For this review, use the dimensioned drawing (mm, ordinates from the lowest corner) and the shaded views. Give positions to 0.01 mm unless a question says otherwise; leave off trailing zeros. Loops run counter-clockwise (first coordinate to the right, second up) from the corner with the lowest first, then second, coordinate; pieces in that order, holes last. Notation, with made-up numbers: M 11.5,-28.75 L 35.5,-28.75 A29 cw 35.5,5.25 Z; hole C 38.5,10.25 d10. An arc over 180 degrees is marked long. Use CSV: the item, a comma, the result in double quotes.
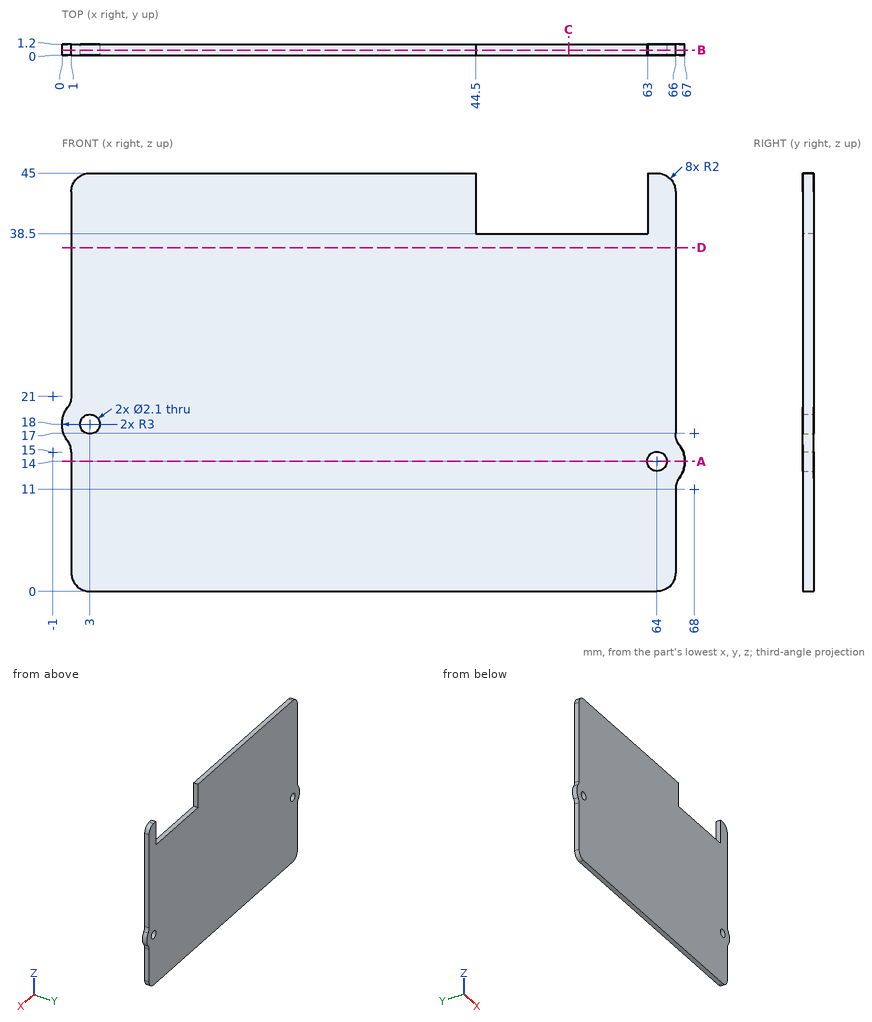
(1) We need section D-D on z = 37. State the section outline as (x, y) points, then the cut area to 3 significant figures.
A:
outline,"M 1,0 L 66,0 L 66,1.2 L 1,1.2 Z"
area,"78.0 mm²"
(2) We need section C-C on x = 54.5. State the section outline as (y, z) points, then the cut area to 3 significant figures.
A:
outline,"M 0,0 L 1.2,0 L 1.2,38.5 L 0,38.5 Z"
area,"46.2 mm²"
(3) Clearance check with a flat-ended pin moving along its axis: P1, Ø1.3, axis at x = 3, z = 18, coming from the +Y side. State where the tip first meets the part, or that it passes through.
A:
P1,"through"
(4) Wall thickness on line 1 along Z through (x, y) = (64, 0.35); line 2 along X through (y, z) = (0.35, 18); line 3 along X through (y, z) = (1.1, 41): over which ranges is each line inside the solid? List them lowest first. Write a range as [from, to].
A:
line 1,"[0, 12.95], [15.05, 45]"
line 2,"[0, 1.95], [4.05, 66]"
line 3,"[1, 44.5], [63, 66]"
(5) We need section B-B on y = 0.55. State the section outline as (x, z) points.
A:
outline,"M 0.6,16.2 A2 cw 1,15 L 1,2 A2 ccw 3,0 L 64,0 A2 ccw 66,2 L 66,11 A2 cw 66.4,12.2 A3 ccw 66.4,15.8 A2 cw 66,17 L 66,43 A2 ccw 64,45 L 63,45 L 63,38.5 L 44.5,38.5 L 44.5,45 L 3,45 A2 ccw 1,43 L 1,21 A2 cw 0.6,19.8 A3 ccw Z; hole C 3,18 d2.1; hole C 64,14 d2.1"
(6) We need section A-A on z = 14. State the section outline as (x, y) points, then the cut area to 3 significant figures.
A:
outline,"M 1,0 L 62.95,0 L 62.95,1.2 L 1,1.2 Z; M 65.05,0 L 67,0 L 67,1.2 L 65.05,1.2 Z"
area,"76.7 mm²"
